Part print with two shaded views. Sizes in mm from the minimum x, y, z corner. A direction names the side the tool comes from. Give positions to 0.01 mm unless a question says otherwise; leave off trailing zeros. Write each loop counter-clockwise with the first axis right and the second up, starting at its lowest first coordinate (ties: lowest second). Pieces come first, ordered by that corner, then holes.
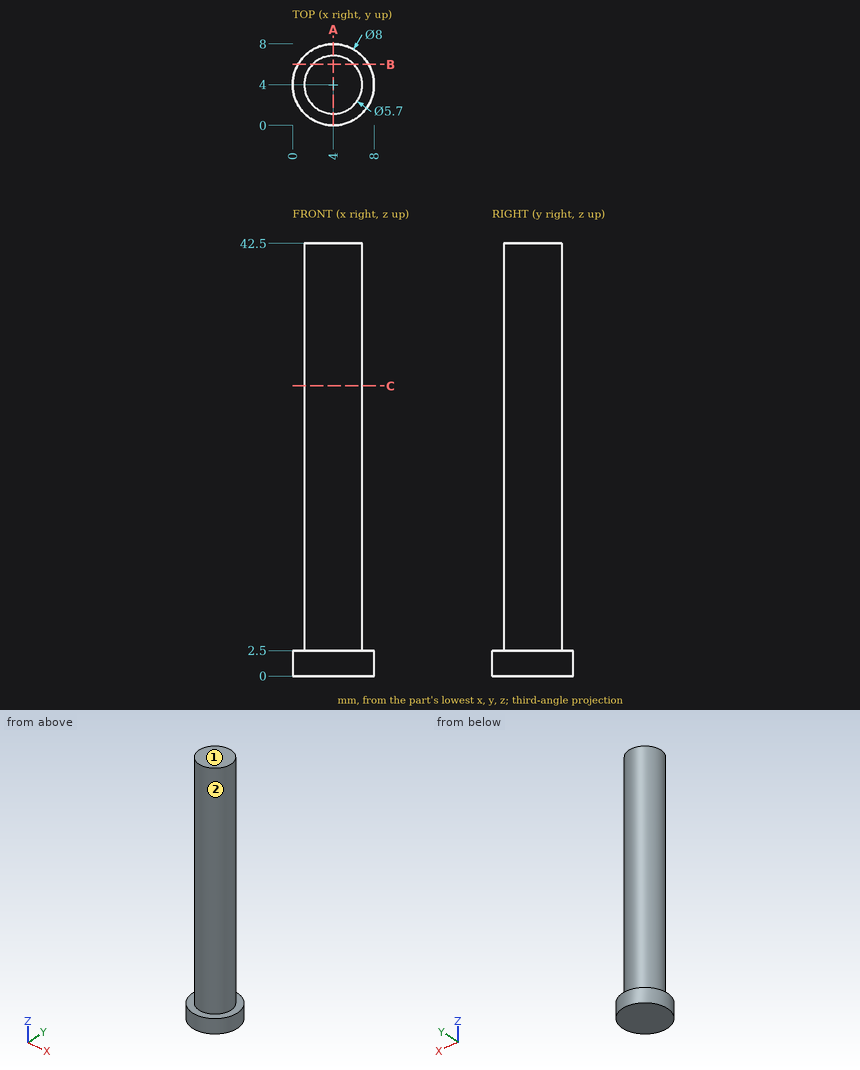
1) Flat gauge pins, fed straight in: P1, Ø4, axis at y = 3.5, z = 23.5, coming from the -X side; P2, Ø1, axis at x = 4.5, z = 37, coming from the -Y side; P3, Ø4, axis at y = 6, z = 23, coming from the +X side. Where does each tip first touch, or does it go through?
Check result:
P1: stops at x = 1.15
P2: stops at y = 1.15
P3: stops at x = 6.85
2) Saw through at C-C (z = 28.5). Write the cut outline in (x, y), and give its area (3 significant figures).
Check result:
outline: circle Ø5.7 at (4, 4)
area: 25.5 mm2
3) Saw through at A-A (x = 4). Write the cut outline in (y, z), and give its area (3 significant figures).
Check result:
outline: (0, 0) - (8, 0) - (8, 2.5) - (6.85, 2.5) - (6.85, 42.5) - (1.15, 42.5) - (1.15, 2.5) - (0, 2.5) - close
area: 248 mm2
4) Saw through at B-B (y = 6). Write the cut outline in (x, z).
Check result:
outline: (0.54, 0) - (7.46, 0) - (7.46, 2.5) - (6.03, 2.5) - (6.03, 42.5) - (1.97, 42.5) - (1.97, 2.5) - (0.54, 2.5) - close
5) 3-axis set-ups, long thin cutter, end or side, ignore diameter. For the marked faces 1 and 2: which of +Z, -Z, +X, -X, +Y, -Y reach the whole face in a straight line?
Check result:
face 1: +Z, +X, -X, +Y, -Y
face 2: +Z
6) Drill centre lines: L1, parallel to Y at x = 4, z = 27.5; L2, parallel to Z at x = 2.5, y = 0.75; L3, parallel to Y at x = 6.5, z = 29. Where is each one in solid material? Low to high.
Check result:
L1: y = 1.15 to 6.85
L2: z = 0 to 2.5
L3: y = 2.63 to 5.37
